Could you check a few things on this model? Use its own coordinates, in mm. Face numbers are marked on the shaded views. A direction names the side the tool comes from. Coordinates: 2 decimals unless noted, no trailing zeros. Loops run counter-clockwise (first coordinate to the right, second up) from the corner with the lowest first, then second, coordinate; pieces in that order, holes last. Notation, with made-up numbers: (23.5, 58) - (34.5, 58) arc R24 ccw to (34.5, 76) - close; hole circle Ø1 at (7, 12.5). An arc over 180 degrees is marked (long way). One line per item, written item: value. Start each with the question number.
(1) If we section it at A-A on z = 0: Write out the boundary of the cut face in (x, y), then the cut area to 3 significant figures.
(2) On a 3-axis mill with a long thin cutter (end or side, diameter ignored), from which of +Z, -Z, +X, -X, +Y, -Y can I reach the whole of each face in a straight line? I mean the marked faces 4, 5 and 6. Say none if no direction works.
(3) If we mould it in two halves opening along X, with no side actions, what happens to the marked faces 1, 2 and 3? For each: pulls with the +X half, pulls with the -X half, needs draft (parallel to the pull), parting line crosses it, or undercut.
(4) If we section it at B-B on y = -4.25: Write out the boundary of the cut face in (x, z).
(5) If I drill on line 1 along Z through (x, y) = (0.15, 0.5); line 2 along Z through (x, y) = (0.4, -5.25); line 3 along Y through (x, z) = (1.55, 1.05), over which ranges is the centre line in solid material (lowest first)? Write a range as from..to.
(6) I'm going to push flat-ended pins straight in: P1, Ø3, axis at x = -2.5, z = -1.5, coming from the -Y side; P2, Ø1.7, axis at x = 1, z = -1, coming from the -Y side. Where does each tip first touch, or does it pass through?
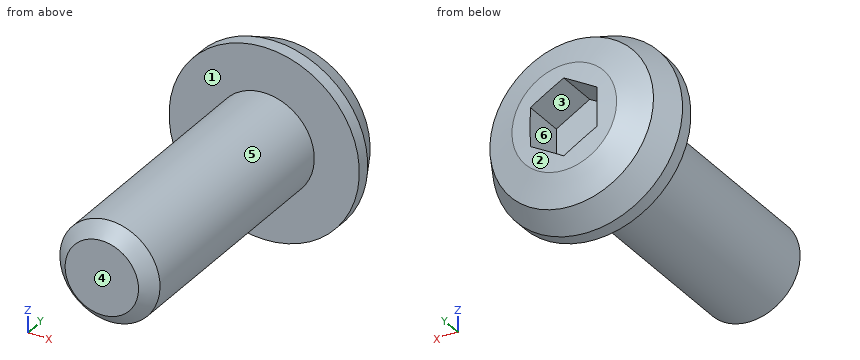
```python
from build123d import *

# Parameters (mm, degrees)
CUT_EXTRUDE1_DEPTH = 1.35


with BuildPart() as part:
    # Sketch1 → Revolve1 (revolve)
    with BuildSketch(Plane.XY, mode=Mode.PRIVATE) as revolve1_sk:
        Polygon((0, -8), (1.1, -8), (1.5, -7.6), (1.5, 0), (2.85, 0), (2.85, 0.4125), (2.451, 1.188), (1.5675, 1.551), (0, 1.65), align=None)
    revolve(revolve1_sk.sketch.rotate(Axis((0, -10, 0), (0, 1, 0)), 90), axis=Axis((0, -10, 0), (0, 1, 0)))

    # Sketch2 → Cut-Extrude1 (cut)
    with BuildSketch(Plane(origin=(0, 1.65, 0), x_dir=(1, 0, 0), z_dir=(0, 1, 0))):
        Polygon((1, -0.577350269), (0, -1.154700538), (-1, -0.577350269), (-1, 0.577350269), (0, 1.154700538), (1, 0.577350269), align=None)
    extrude(amount=-CUT_EXTRUDE1_DEPTH, mode=Mode.SUBTRACT)


solid = part.part
```
Values:
1. outline: (-2.85, 0) - (-1.5, 0) - (-1.5, -7.6) - (-1.1, -8) - (1.1, -8) - (1.5, -7.6) - (1.5, 0) - (2.85, 0) - (2.85, 0.41) - (2.45, 1.19) - (1.57, 1.55) - (1, 1.59) - (1, 0.3) - (-1, 0.3) - (-1, 1.59) - (-1.57, 1.55) - (-2.45, 1.19) - (-2.85, 0.41) - close
1. area: 29.3 mm2
2. face 4: +Z, -Z, +X, -X, -Y
2. face 5: -Y
2. face 6: +Y
3. face 1: needs draft
3. face 2: parting line crosses it
3. face 3: undercut
4. outline: circle Ø3 at (0, 0)
5. line 1: z = -2.8..-1.07, 1.07..2.8
5. line 2: z = -1.45..1.45
5. line 3: y = 0..1.43
6. P1: stops at y = -7.68
6. P2: stops at y = -8
